Could you check a few things on this model? Use its own coordinates, in mm. A direction names the side the tool comes from. Round coordinates to 2 decimals unless told otherwise and drop trailing zeros. Loops run counter-clockwise (first coordinate to the right, second up) from the corner with the lowest first, then second, coordinate; pieces in that order, holes last. Notation, with made-up numbers: M -26,-19.75 L 32,-19.75 A8 cw 32,-4.75 Z; hole C 84,27.5 d1. An arc over 180 degrees is marked long. Return JSON: item names as keys, results as strings. Group by question number.
```python
from build123d import *

# Parameters (mm, degrees)
SKETCH1_W           = 55.6
SKETCH1_H           = 35
SKETCH1_W_2         = 45.6
SKETCH1_H_2         = 25
BOSS_EXTRUDE1_DEPTH = 52
SKETCH2_W           = 45.6
SKETCH2_H           = 42
CUT_EXTRUDE1_DEPTH  = 5
SKETCH3_R           = 1.6
SKETCH3_W           = 40
SKETCH3_H           = 20.5
CUT_EXTRUDE2_DEPTH  = 5


with BuildPart() as part:
    # Sketch1 → Boss-Extrude1 (new body)
    with BuildSketch(Plane(origin=(0, 0, 0), x_dir=(1, 0, 0), z_dir=(0, 1, 0))):
        with Locations((27.8, -17.5)):
            Rectangle(SKETCH1_W, SKETCH1_H)
        with Locations((27.8, -17.5)):
            Rectangle(SKETCH1_W_2, SKETCH1_H_2, mode=Mode.SUBTRACT)
    extrude(amount=BOSS_EXTRUDE1_DEPTH)

    # Sketch2 → Cut-Extrude1 (cut)
    with BuildSketch(Plane.XY.offset(35)):
        with Locations((27.8, 26)):
            Rectangle(SKETCH2_W, SKETCH2_H)
    extrude(amount=-CUT_EXTRUDE1_DEPTH, mode=Mode.SUBTRACT)

    # Sketch3 → Cut-Extrude2 (cut)
    with BuildSketch(Plane.XY.offset(35)):
        with Locations((51.1, 20.2)):
            Circle(SKETCH3_R)
        with Locations((51.1, 10.3)):
            Circle(SKETCH3_R)
        with Locations((2.5, 10.3)):
            Circle(SKETCH3_R)
        with Locations((2.5, 20.2)):
            Circle(SKETCH3_R)
        with Locations((26.8, 15.25)):
            Rectangle(SKETCH3_W, SKETCH3_H)
    extrude(amount=-CUT_EXTRUDE2_DEPTH, mode=Mode.SUBTRACT)


solid = part.part
```
1. If we section it at D-D, the plane y = 48.5: Please give me the cut outline in (x, z), then the cut area to 3 significant figures.
2. We'd pull the mould along X, two halves only. Please class faces 4 (the face through (52.7, 10.3, 32.5)), 5 (the face through (27, 0, 33)), 6 (the face through (27, 5, 33)), 7 (the face through (0, 26, 18)): +X half, -X half, draft (parallel to the pull), parting line (faces both ways), or undercut.
3. I'm going to push flat-ended pins straight in: pin 1 Ø1 at (x, y) = (2, 10) entering from +Z; pin 2 Ø4 at (x, y) = (24, 14) entering from +Z. Where does each tip first touch, or does it pass through?
4. On a 3-axis mill with a long thin cutter (end or side, diameter ignored), from which of +Z, -Z, +X, -X, +Y, -Y can I reach the whole of each face in a straight line? I mean faces 1 (the face through (5, 26, 20)), 2 (the face through (52.7, 20.2, 32.5)), 3 (the face through (27, 2, 30)). Say none if no direction works.
5. If we section it at A-A, the plane z = 13: Please give me the cut outline in (x, y).
6. If we section it at C-C, the plane x = 16: Please give me the cut outline in (y, z).
7. If we section it at B-B, the plane y = 10.3: Please give me the cut outline in (x, z).
8. I need wall thicknesses on probe 1 along Y at (x, z) = (2.5, 32.9); probe 2 along X at (y, z) = (33, 16); probe 3 along X at (y, z) = (20, 33). Which ranges of each line are inside material? Lowest first, please.
Geometry results:
{
 "1": {"outline": "M 0,0 L 55.6,0 L 55.6,35 L 0,35 Z; hole M 5,5 L 50.6,5 L 50.6,30 L 5,30 Z", "area": "806 mm^2"},
 "2": {"face 4": "undercut", "face 5": "draft", "face 6": "undercut", "face 7": "-X half"},
 "3": {"pin 1": "z = 30", "pin 2": "z = 5"},
 "4": {"face 1": "none", "face 2": "+Z", "face 3": "+Y, -Y"},
 "5": {"outline": "M 0,0 L 5,0 L 5,52 L 0,52 Z; M 50.6,0 L 55.6,0 L 55.6,52 L 50.6,52 Z"},
 "6": {"outline": "M 0,0 L 52,0 L 52,5 L 0,5 Z; M 0,30 L 5,30 L 5,35 L 0,35 Z; M 47,30 L 52,30 L 52,35 L 47,35 Z"},
 "7": {"outline": "M 0,0 L 55.6,0 L 55.6,35 L 52.7,35 L 52.7,30 L 50.6,30 L 50.6,5 L 5,5 L 5,35 L 4.1,35 L 4.1,30 L 0.9,30 L 0.9,35 L 0,35 Z"},
 "8": {"probe 1": "0 to 8.7, 11.9 to 18.6, 21.8 to 52", "probe 2": "0 to 5, 50.6 to 55.6", "probe 3": "0 to 0.91, 4.09 to 5, 52.69 to 55.6"}
}
